Model file for the job. Use its own axes, mm. A direction names the side the tool comes from. Coordinates: 2 decimals unless noted, no trailing zeros. Loops run counter-clockwise (first coordinate to the right, second up) from the corner with the lowest first, then second, coordinate; pieces in that order, holes last.
Autodesk Inventor part; units mm, degrees
ref_plane "YZ Plane" through (0, 0, 0) normal (1, 0, 0) x (0, 1, 0)
ref_plane "XZ Plane" through (0, 0, 0) normal (0, 1, 0) x (-1, 0, 0)
ref_plane "XY Plane" through (0, 0, 0) normal (0, 0, 1) x (1, 0, 0)
sketch "Sketch1" plane through (0, 0, 0) normal (0, 1, 0) x (-1, 0, 0)
  line L0 (0, 0) -> (0, -48.498)
  line L1 (0, 0) -> (25.5001, 14.7225)
  line L2 (0, 0) -> (29.445, 0) construction
  line L3 (0, -48.498) -> (25.5001, -63.2205)
  line L4 (0, -48.498) -> (29.445, -48.498) construction
  line L5 (25.5001, -63.2205) -> (23.5001, -66.6846)
  line L6 (0, -46.9861) -> (-4, -46.9861)
  line L7 (-4, -46.9861) -> (-4, -50.8074)
  line L8 (-4, -50.8074) -> (23.5001, -66.6846)
  line L9 (1.1556, 0.6672) -> (-0.8444, 4.1313)
  line L10 (-0.8444, 4.1313) -> (-4, 2.3094)
  line L11 (-4, 2.3094) -> (-4, -46.9861)
  line L12 (-0.8444, 4.1313) -> (23.5001, 18.1866)
  line L13 (23.5001, 18.1866) -> (25.5001, 14.7225)
  dimension "d0" = 48.498
  dimension "d1" = 29.445
  dimension "d2" = 30
  dimension "d3" = 29.445
  dimension "d4" = 30
  dimension "d5" = 4
  dimension "d6" = 4
  dimension "d7" = 4
extrude "Extrusion1" add sketch "Sketch1" along normal blind 40
sketch "Sketch2" plane through (0, 0, 0) normal (0, -1, 0) x (1, 0, 0)
  line L0 (0, 0) -> (-25.5001, 14.7225)
  line L1 (-25.5001, 14.7225) -> (-23.1946, 18.7157)
  line L2 (-25.5001, 14.7225) -> (-23.5001, 18.1866)
  line L3 (-23.1946, 18.7157) -> (-25.5001, 14.7225)
  line L4 (-25.5001, 14.7225) -> (-21.5069, 12.417)
  line L5 (-21.5069, 12.417) -> (-17.5069, 19.3452)
  circle A0 centre (-17.5069, 19.3452) radius 1.75
  circle A1 centre (-17.5069, 19.3452) radius 3.5
  line L6 (-20.538, 21.0952) -> (-22.538, 17.6311)
  line L7 (-23.5001, 18.1866) -> (4, 2.3094)
  line L8 (-14.4758, 17.5952) -> (-16.4758, 14.1311)
  dimension "d10" = 4.611
  dimension "d11" = 4.611
  dimension "d12" = 8
  dimension "d13" = 3.5
  dimension "d14" = 7
extrude "Extrusion2" add sketch "Sketch2" against normal blind 3 contours A1
sketch "Sketch3" plane through (-17.5069, 3, 19.3452) normal (0, 1, 0) x (1, 0, 0)
  circle A0 centre (0, 0) radius 1.75
  line L0 (0, 0) -> (-2, 3.4641)
  line L1 (-5.9932, 1.1586) -> (21.5069, 17.0358)
  line L2 (-2, 3.4641) -> (-5.0311, 1.7141)
  line L3 (-5.0311, 1.7141) -> (-3.0311, -1.75)
  circle A1 centre (0, 0) radius 3.5
  line L4 (-2, 3.4641) -> (1.0311, 5.2141)
  line L5 (1.0311, 5.2141) -> (2.9919, 1.8179)
  line L6 (2.9919, 1.8179) -> (1.5256, 0.9713)
  line L7 (1.5256, 0.9713) -> (0.9971, 2.6723)
  line L8 (0.9971, 2.6723) -> (-1.1427, 2.5009)
  line L9 (-1.1427, 2.5009) -> (-2.2108, 1.3125)
  line L10 (-2.2108, 1.3125) -> (-2.3481, -0.99)
  line L11 (-2.3481, -0.99) -> (-3.0311, -1.75)
  point P0 (17.5069, 19.3452)
  dimension "d17" = 3.5
  dimension "d18" = 3.5
extrude "Extrusion3" add sketch "Sketch3" against normal blind 3 contours L9 L10 L11 A1 L0 | L0 A1 L6 L7 L8 L9 | A1 L3 L1 L0 | L0 L1 L5 A1
sketch "Sketch4" plane through (0, 0, 0) normal (0, -1, 0) x (1, 0, 0)
  line L0 (-23.5001, -66.6846) -> (-25.5001, -63.2205)
  line L1 (-23.5001, -66.6846) -> (-21.1946, -70.6778)
  line L2 (-21.1946, -70.6778) -> (-23.5001, -66.6846)
  line L3 (-25.5001, -63.2205) -> (0, -48.498)
  line L4 (-25.5001, -63.2205) -> (-21.5069, -60.915)
  line L5 (-21.5069, -60.915) -> (-17.5069, -67.8432)
  circle A0 centre (-17.5069, -67.8432) radius 1.75
  circle A1 centre (-17.5069, -67.8432) radius 3.5
  line L6 (-19.5069, -64.3791) -> (-22.538, -66.1291)
  line L7 (4, -50.8074) -> (-23.5001, -66.6846)
  line L8 (-22.538, -66.1291) -> (-20.538, -69.5932)
  line L9 (-19.5069, -64.3791) -> (-16.4758, -62.6291)
  line L10 (-16.4758, -62.6291) -> (-14.4758, -66.0932)
  point P0 (0, 0)
  dimension "d21" = 4.611
  dimension "d22" = 4.611
  dimension "d23" = 8
  dimension "d24" = 3.5
  dimension "d25" = 7
  dimension "d26" = 3.5
  dimension "d27" = 3.5
extrude "Extrusion4" add sketch "Sketch4" against normal blind 3 contours L6 L5 A1 L8 | L7 L10 A1 L5 | A1
sketch "Sketch5" plane through (0, 0, 0) normal (0, -1, 0) x (1, 0, 0)
  line L0 (0, -48.498) -> (0, 0)
  line L1 (0, -24.249) -> (8, -24.249)
  circle A0 centre (8, -24.249) radius 1.75
  circle A1 centre (8, -24.249) radius 3.5
  line L2 (4, 2.3094) -> (4, -50.8074)
  line L3 (4, -24.249) -> (4, -27.749)
  line L4 (4, -27.749) -> (8, -27.749)
  line L5 (4, -24.249) -> (4, -20.749)
  line L6 (4, -20.749) -> (8, -20.749)
  dimension "d30" = 8
  dimension "d31" = 3.5
  dimension "d32" = 7
extrude "Extrusion5" add sketch "Sketch5" against normal blind 3
sketch "Sketch6" plane through (0, 40, 0) normal (0, 1, 0) x (1, 0, 0)
  line L0 (4, -2.3094) -> (4, 50.8074)
  line L1 (4, 24.249) -> (8, 24.249)
  circle A0 centre (8, 24.249) radius 1.75
  circle A1 centre (8, 24.249) radius 3.5
  line L2 (4, 27.749) -> (4, 50.8074)
  line L3 (4, 24.249) -> (4, 27.749)
  line L4 (8, 27.749) -> (4, 27.749)
  line L5 (4, 27.749) -> (8, 27.749)
  line L6 (4, 24.249) -> (4, 20.749)
  line L7 (4, 20.749) -> (8, 20.749)
  line L8 (4, 20.749) -> (8, 20.749)
  point P0 (0, 0)
  dimension "d35" = 4
  dimension "d36" = 3.5
  dimension "d37" = 7
extrude "Extrusion6" add sketch "Sketch6" against normal blind 3
properties part number "Capture Zone3"
Q1. Slice it at C-C (z = -58). List the corners of the cut face in (x, y).
Answers:
outline: (-16.46, 0) - (-8.46, 0) - (-8.46, 40) - (-16.46, 40) - close
Q2. Which spindle directions (+Z, -Z, +X, -X, +Y, -Y) get a long thin tool onto all of the face, cutting with end or side? Do faces 5 (the flat face through (-12.572, 19.72, 7.258)), 6 (the flat face through (6, 39, -27.749)), 7 (the flat face through (6, 37, -24)), 8 (the flat face through (-15.509, 1.521, 15.805)), 9 (the flat face through (-19.3, 3, -66.9)). Say none if no direction does.
Answers:
face 5: -X, +Y, -Y
face 6: -Z, +X, +Y, -Y
face 7: +Z, -Z, +X
face 8: +X, +Y, -Y
face 9: -Z, +X, +Y
Q3. Slice it at B-B (z = -18). List the corners of the cut face in (x, y).
Answers:
outline: (0, 0) - (4, 0) - (4, 40) - (0, 40) - close
Q4. Flat gauge pins, fed straight in: P1, Ø5.5, axis at x = 7, z = -25.5, coming from the -Y side; P2, Ø6, axis at y = 33, z = -52, coming from the -X side; P3, Ø12, axis at y = 20, z = -37.5, coming from the +X side; P4, Ø3, axis at x = -17.51, z = -67.84, coming from the +Y side. Where does each tip first touch, or does it go through?
Answers:
P1: stops at y = 0
P2: stops at x = -11.26
P3: stops at x = 4
P4: passes through
Q5. Drill centre lines: line 1 (Z direction, x = 8, y = 1.9); line 2 (Y direction, x = 6, z = -22.5); line 3 (Y direction, x = -15.5, z = -65.5). Where is each one in solid material? Low to high.
Answers:
line 1: z = -27.75 to -26, -22.5 to -20.75
line 2: y = 0 to 3, 37 to 40
line 3: y = 0 to 3
Q6. Mould opens along X. For faces 1 (the flat face through (-24.514, 19.72, -64.928)), 2 (the flat face through (6, 1, -27.749)), 3 (the cylindrical face through (-17.89, 1.48, -69.55)), 4 (the cylindrical face through (-17.73, 1.48, 21.08)) say: +X half, -X half, draft (parallel to the pull), parting line (faces both ways), or undercut.
Answers:
face 1: -X half
face 2: draft
face 3: undercut
face 4: undercut
Q7. Slice it at A-A (y = 4). List the corners of the cut face in (x, z).
Answers:
outline: (-25.5, -63.22) - (-23.5, -66.68) - (4, -50.81) - (4, 2.31) - (0.84, 4.13) - (-23.5, 18.19) - (-25.5, 14.72) - (0, 0) - (0, -48.5) - close
